```python
from build123d import *

# Parameters (mm, degrees)
F0_W     = 60
F0_H     = 70
F0_R     = 2
F1_DEPTH = 30
F2_DEPTH = 32
F3_R     = 5


with BuildPart() as f1:
    # F0 (on Front) → F1 (new body)
    with BuildSketch(Plane.XZ):
        Rectangle(F0_W, F0_H)
        with Locations((-15, -23.889102)):
            Circle(F0_R, mode=Mode.SUBTRACT)
        with Locations((-5, -23.889102)):
            Circle(F0_R, mode=Mode.SUBTRACT)
        with Locations((5, -23.889102)):
            Circle(F0_R, mode=Mode.SUBTRACT)
        with Locations((15, -24.129193)):
            Circle(F0_R, mode=Mode.SUBTRACT)
    extrude(amount=F1_DEPTH)

    # F0 (on Front) → F2 (join)
    with BuildSketch(Plane.XZ):
        with Locations((15, -24.129193)):
            Circle(F0_R)
        with Locations((5, -23.889102)):
            Circle(F0_R)
        with Locations((-5, -23.889102)):
            Circle(F0_R)
        with Locations((-15, -23.889102)):
            Circle(F0_R)
    extrude(amount=F2_DEPTH)

    # F3
    f3_edges = [f1.edges().sort_by_distance(p)[0] for p in [
        (-30, -15, 35),
        (0, 0, 35),
        (0, -30, 35),
        (30, -15, 35),
        (30, -30, 0),
        (-30, -30, 0),
        (-30, 0, 0),
        (30, 0, 0),
        (0, 0, -35),
        (0, -30, -35),
        (30, -15, -35),
        (-30, -15, -35),
    ]]
    fillet(f3_edges, radius=F3_R)


solid = f1.part
```
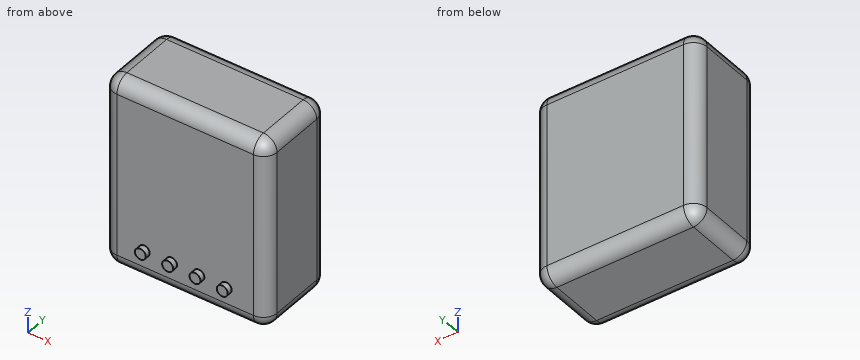
CAD build for the part. Positions are in the model's coordinates, mm. Coordinates: 2 decimals unless noted, no trailing zeros. Order: outer loops, then holes, each group sorted by start corner. A loop starts at its lowest first (then second) coordinate and runs counter-clockwise, first axis right, second up. Notation, with made-up numbers: (-35.5, 35.5) - (-8.5, 35.5) arc R18 ccw to (-8.5, 49.5) - close; hole circle Ø9 at (-3, 74.25). An arc over 180 degrees is marked (long way). Use a Markdown table: item, result. Add a question column.
(1) Saw through at C-C (x = 5). Give the cut face in (y, z).
(2) Drill centre lines: line 1 along Y through (x, z) = (-14, -7); line 2 along Z through (x, y) = (-9, -25.5); line 3 along Z through (x, y) = (6, -27). Where is each one in solid material? Low to high. Write a range as [from, to].
(3) Saw through at B-B (y = -2). Give the cut face in (x, z), then the cut area to 3 significant figures.
(4) Saw through at A-A (z = 28). Give the cut face in (x, y).
Solved:
| question | item | result |
|---|---|---|
| 1 | outline | (-32, -25.89) - (-30, -25.89) - (-30, -30) arc R5 ccw to (-25, -35) - (-5, -35) arc R5 ccw to (0, -30) - (0, 30) arc R5 ccw to (-5, 35) - (-25, 35) arc R5 ccw to (-30, 30) - (-30, -21.89) - (-32, -21.89) - close |
| 2 | line 1 | y = [-30, 0] |
| 2 | line 2 | z = [-34.97, 34.97] |
| 2 | line 3 | z = [-34.58, 34.58] |
| 3 | outline | (-29, -30) arc R4 ccw to (-25, -34) - (25, -34) arc R4 ccw to (29, -30) - (29, 30) arc R4 ccw to (25, 34) - (-25, 34) arc R4 ccw to (-29, 30) - close |
| 3 | area | 3,930 mm² |
| 4 | outline | (-30, -25) arc R5 ccw to (-25, -30) - (25, -30) arc R5 ccw to (30, -25) - (30, -5) arc R5 ccw to (25, 0) - (-25, 0) arc R5 ccw to (-30, -5) - close |
